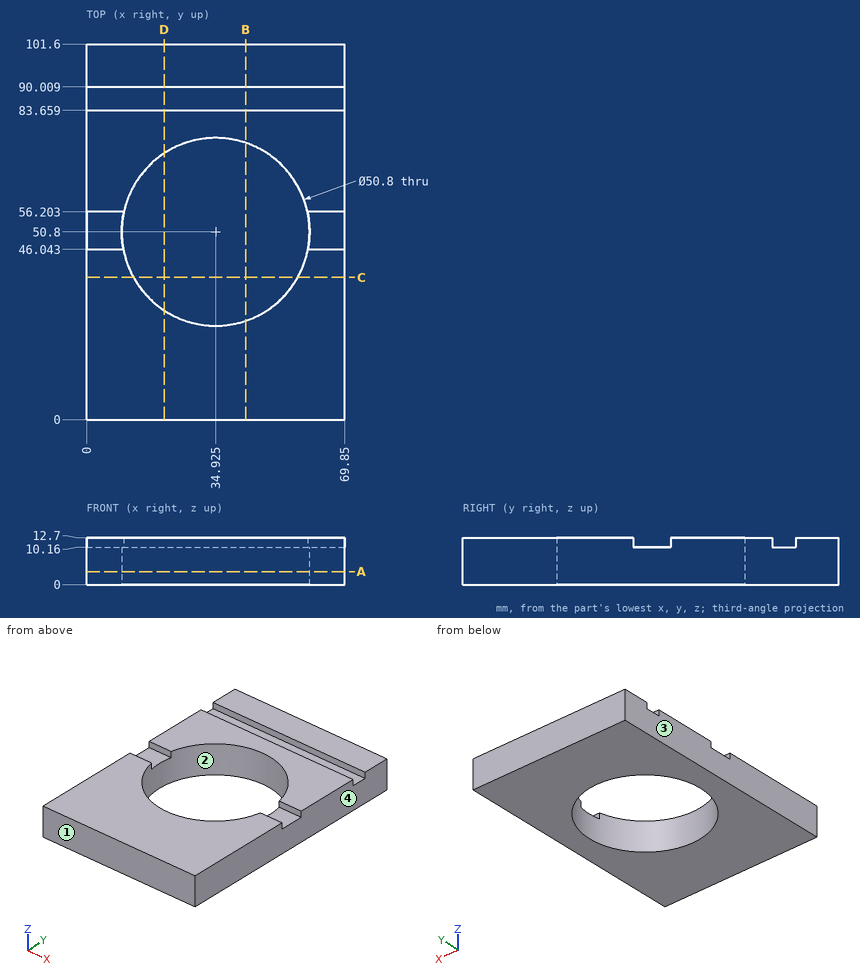
Check sheet for the drawn part. Datum: minimum x, y, z corner. Units: mm. Give positions to 0.01 mm unless a question says otherwise; leave off trailing zeros. Write each loop counter-clockwise with the first axis right and the second up, starting at its lowest first coordinate (ties: lowest second). Pieces come first, ordered by that corner, then holes. Notation, with made-up numbers: (86, -4.75) -> (110, -4.75) arc R9 cw to (110, 5.25) -> close; hole circle Ø5 at (62.25, 19). An arc over 180 degrees is marked (long way). Use one line per item in the form item = value. Start each with the question number.
1. Mould release check, pull along X, two halves, no side actions. Record for the marked faces 1, 2, 3 and 4: pulls with the +X half, pulls with the -X half, needs draft (parallel to the pull), parting line crosses it, or undercut.
2. Section check D-D (x = 21). Record the cut outline in (y, z), and give its area (3 significant figures).
3. Thickness scan on line 1 along Y through (x, z) = (61, 12); line 2 along X through (y, z) = (50.8, 8) (3 decimals); line 3 along Y through (x, z) = (20, 10.25). Record the ranges inside material, lowest first. Write a range as from..to.
4. Go/stop test with a flat-tipped pin: P1, Ø5, axis at x = 63, y = 50, coming from the +Z side. Record where the tip stops, or that it passes through.
5. Section check A-A (z = 3.5). Record the cut outline in (x, y) (3 decimals), and give its area (3 significant figures).
6. Section check C-C (y = 38.5). Record the cut outline in (x, z).
7. Section check B-B (x = 43). Record the cut outline in (y, z).
Conclusion:
q1.face_1 = needs draft
q1.face_2 = undercut
q1.face_3 = pulls with the -X half
q1.face_4 = pulls with the +X half
q2.outline = (0, 0) -> (29.56, 0) -> (29.56, 12.7) -> (0, 12.7) -> close; (72.04, 0) -> (101.6, 0) -> (101.6, 12.7) -> (90.01, 12.7) -> (90.01, 10.16) -> (83.66, 10.16) -> (83.66, 12.7) -> (72.04, 12.7) -> close
q2.area = 735 mm²
q3.line_1 = 0..46.04, 56.2..83.66, 90.01..101.6
q3.line_2 = 0..9.525, 60.325..69.85
q3.line_3 = 0..30.25, 71.35..83.66, 90.01..101.6
q4.P1 = 10.16
q5.outline = (0, 0) -> (69.85, 0) -> (69.85, 101.6) -> (0, 101.6) -> close; hole circle Ø50.8 at (34.925, 50.8)
q5.area = 5,070 mm²
q6.outline = (0, 0) -> (12.7, 0) -> (12.7, 12.7) -> (0, 12.7) -> close; (57.15, 0) -> (69.85, 0) -> (69.85, 12.7) -> (57.15, 12.7) -> close
q7.outline = (0, 0) -> (26.72, 0) -> (26.72, 12.7) -> (0, 12.7) -> close; (74.88, 0) -> (101.6, 0) -> (101.6, 12.7) -> (90.01, 12.7) -> (90.01, 10.16) -> (83.66, 10.16) -> (83.66, 12.7) -> (74.88, 12.7) -> close
